from build123d import *

# Parameters (mm, degrees)
BOSS_EXTRUDE1_DEPTH = 18.25625
SKETCH2_R           = 1.5875
CUT_EXTRUDE1_DEPTH  = 1092.171116308
SKETCH3_R           = 1.5875
CUT_EXTRUDE2_DEPTH  = 1092.171116308


with BuildPart() as part:
    # Sketch1 → Boss-Extrude1 (new body)
    with BuildSketch(Plane.XY):
        with BuildLine():
            Line((0, 990.6), (0, 0))
            Line((0, 0), (457.201, 0))
            Line((457.201, 0), (457.201, 13.862038208))
            ThreePointArc((457.201, 13.862038208), (232.767577124, 176.628269142), (124.367415652, 431.8))
            Line((124.367415652, 431.8), (50.8, 990.6))
            Line((50.8, 990.6), (0, 990.6))
        make_face()
    extrude(amount=BOSS_EXTRUDE1_DEPTH)

    # Sketch2 → Cut-Extrude1 (cut, through all)
    with BuildSketch(Plane.XY.offset(18.25625)):
        with Locations((12.7, 977.9)):
            Circle(SKETCH2_R)
        with Locations((38.1, 977.9)):
            Circle(SKETCH2_R)
        with Locations((12.7, 901.7)):
            Circle(SKETCH2_R)
        with Locations((38.1, 901.7)):
            Circle(SKETCH2_R)
        with Locations((12.7, 609.6)):
            Circle(SKETCH2_R)
        with Locations((38.1, 609.6)):
            Circle(SKETCH2_R)
        with Locations((12.7, 685.8)):
            Circle(SKETCH2_R)
        with Locations((38.1, 685.8)):
            Circle(SKETCH2_R)
        with Locations((12.7, 254)):
            Circle(SKETCH2_R)
        with Locations((38.1, 254)):
            Circle(SKETCH2_R)
        with Locations((12.7, 330.2)):
            Circle(SKETCH2_R)
        with Locations((38.1, 330.2)):
            Circle(SKETCH2_R)
        with Locations((12.7, 38.1)):
            Circle(SKETCH2_R)
        with Locations((12.7, 12.7)):
            Circle(SKETCH2_R)
        with Locations((88.9, 38.1)):
            Circle(SKETCH2_R)
        with Locations((88.9, 12.7)):
            Circle(SKETCH2_R)
        with Locations((241.3, 38.1)):
            Circle(SKETCH2_R)
        with Locations((317.5, 38.1)):
            Circle(SKETCH2_R)
        with Locations((241.3, 12.7)):
            Circle(SKETCH2_R)
        with Locations((317.5, 12.7)):
            Circle(SKETCH2_R)
    extrude(amount=-CUT_EXTRUDE1_DEPTH, mode=Mode.SUBTRACT)

    # Sketch3 → Cut-Extrude2 (cut, through all)
    with BuildSketch(Plane.XY.offset(18.25625)):
        with Locations((64.74219971, 787.4)):
            Circle(SKETCH3_R)
        with Locations((54.710279394, 863.6)):
            Circle(SKETCH3_R)
    extrude(amount=-CUT_EXTRUDE2_DEPTH, mode=Mode.SUBTRACT)


solid = part.part
Can you work these out from the model? Positions are in its coordinate system, mm. Coordinates: 2 decimals unless noted, no trailing zeros. Write each loop counter-clockwise with the first axis right and the second up, starting at its lowest first coordinate (ties: lowest second). Pieces come first, ordered by that corner, then holes. Notation, with made-up numbers: (89, 2) -> (147, 2) arc R10 cw to (147, 14) -> close; hole circle Ø2 at (59, -26.75). An arc over 180 degrees is marked (long way). Write each question's results on one line, items separated by ' | '. Start each with the question number.
Item 1: If we section it at B-B, the plane x = 262.5: Write out the boundary of the cut face in (y, z).
Item 2: If we section it at C-C, the plane y = 278: Write out the boundary of the cut face in (x, z), and give its area (3 significant figures).
Item 3: Please list where these lines run through material, in increasing order: probe 1 along X at (y, z) = (685.8, 8); probe 2 along Y at (x, z) = (216, 6); probe 3 along Y at (x, z) = (405, 6.75).
Item 4: I'm going to push flat-ended pins straight in: P1, Ø5, axis at y = 853.5, z = 12.5, coming from the +X side; P2, Ø3, axis at y = 406, z = 8.5, coming from the +X side; P3, Ø10, axis at y = 696.5, z = 16, coming from the +X side. Where does each tip first touch, or does it pass through?
Item 5: If we section it at A-A, the plane z = 15.5: Count the separate pieces of the cut face and the enclosed holes in it, and give its area (3 significant figures).
Answer block:
1) outline: (0, 0) -> (142.47, 0) -> (142.47, 18.26) -> (0, 18.26) -> close
2) outline: (0, 0) -> (169.63, 0) -> (169.63, 18.26) -> (0, 18.26) -> close | area: 3,100 mm²
3) probe 1: 0 to 11.11, 14.29 to 36.51, 39.69 to 90.93 | probe 2: 0 to 198.89 | probe 3: 0 to 36.65
4) P1: x = 69.18 | P2: x = 128.71 | P3: x = 90.18
5) separate pieces: 1 | enclosed holes: 22 | area: 150,000 mm²
